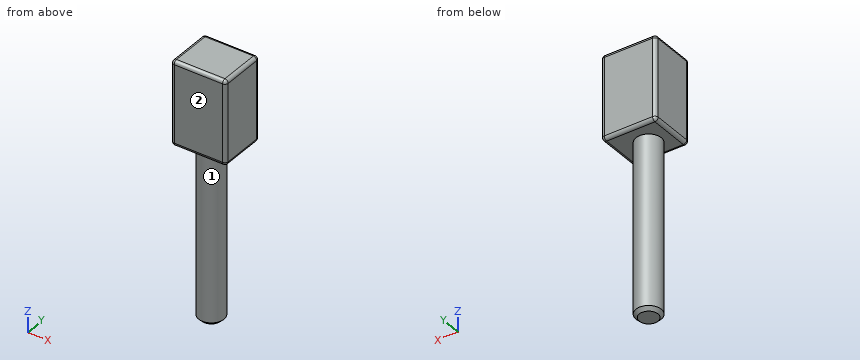
from build123d import *

# Parameters (mm, degrees)
F0_W     = 83.694592
F0_H     = 71.509171
F1_DEPTH = 128.27
F2_R     = 5.08
F3_R     = 19.259612
F4_DEPTH = 263.398
F5_SIZE  = 5.08


with BuildPart() as f1:
    # F0 (on Top) → F1 (new body)
    with BuildSketch(Plane.XY):
        with Locations((3.848031, 2.405015)):
            Rectangle(F0_W, F0_H)
    extrude(amount=F1_DEPTH)

    # F2
    f2_edges = [f1.edges().sort_by_distance(p)[0] for p in [
        (45.695327, 38.159601, 64.135),
        (-37.999265, 38.159601, 64.135),
        (3.848031, 38.159601, 0),
        (3.848031, 38.159601, 128.27),
        (3.848031, -33.34957, 128.27),
        (45.695327, 2.405016, 128.27),
        (-37.999265, 2.405016, 128.27),
        (45.695327, -33.34957, 64.135),
        (45.695327, 2.405016, 0),
        (3.848031, -33.34957, 0),
        (-37.999265, 2.405016, 0),
        (-37.999265, -33.34957, 64.135),
    ]]
    fillet(f2_edges, radius=F2_R)

    # F3 (on Top) → F4 (join)
    with BuildSketch(Plane.XY):
        Circle(F3_R)
    extrude(amount=-F4_DEPTH)

    # F5
    f5_edges = [f1.edges().sort_by_distance(p)[0] for p in [
        (-19.259612, 0, -263.398),
    ]]
    chamfer(f5_edges, length=F5_SIZE)


solid = f1.part
Build history of the part. All positions in model axes, mm. Face numbers are marked on the shaded views. A direction names the side the tool comes from. Give positions to 0.01 mm unless a question says otherwise; leave off trailing zeros. Order: outer loops, then holes, each group sorted by start corner. A loop starts at its lowest first (then second) coordinate and runs counter-clockwise, first axis right, second up. Notation, with made-up numbers: M 84,-27.5 L 96,-27.5 A31 cw 96,1.5 Z; hole C -17,-5 d2. An arc over 180 degrees is marked long. Put each result on its own line as item: value.
Item 1: Wall check: probe 1 along Z at (x, y) = (12, -16); probe 2 along Y at (x, z) = (13, -109); probe 3 along X at (y, z) = (0.5, -196). Give the ranges that are in metal, low to high.
Results are:
probe 1: 0 to 128.27
probe 2: -14.21 to 14.21
probe 3: -19.25 to 19.25
Item 2: Cut at A-A on y = 0. Write the cut outline in (x, z).
Results are:
outline: M -38,5.08 A5.08 ccw -32.92,0 L -19.26,0 L -19.26,-258.32 L -14.18,-263.4 L 14.18,-263.4 L 19.26,-258.32 L 19.26,0 L 40.62,0 A5.08 ccw 45.7,5.08 L 45.7,123.19 A5.08 ccw 40.62,128.27 L -32.92,128.27 A5.08 ccw -38,123.19 Z
Item 3: Cut at C-C on x = 27.5. Write the cut outline in (y, z), then the cut area to 3 significant figures.
Results are:
outline: M -33.35,5.08 A5.08 ccw -28.27,0 L 33.08,0 A5.08 ccw 38.16,5.08 L 38.16,123.19 A5.08 ccw 33.08,128.27 L -28.27,128.27 A5.08 ccw -33.35,123.19 Z
area: 9,150 mm2
Item 4: Drop flat-ended pins along their axis: pin 1 Ø4 at (x, y) = (1.5, -20) entering from -Z; pin 2 Ø5 at (y, z) = (-24, -30.5) entering from +X; pin 3 Ø2 at (x, y) = (-9, 15) entering from -Z; pin 4 Ø5 at (x, y) = (36.5, -24) entering from -Z. Give the stop position or say it passes through.
Results are:
pin 1: z = -259.52
pin 2: through
pin 3: z = -261.08
pin 4: z = 0
Item 5: Which spindle directions (+Z, -Z, +X, -X, +Y, -Y) get a long thin tool onto all of the face, cutting with end or side? Do the marked faces 1 and 2. Say none if no direction does.
Results are:
face 1: -Z
face 2: +Z, -Z, +X, -X, -Y
Item 6: Cut at D-D on z = -196.5. Write the cut outline in (x, y), then the cut area to 3 significant figures.
Results are:
outline: C 0,0 d38.52
area: 1,170 mm2
Item 7: Cut at B-B on x = 0. Write the cut outline in (y, z), then the cut area to 3 significant figures.
Results are:
outline: M -33.35,5.08 A5.08 ccw -28.27,0 L -19.26,0 L -19.26,-258.32 L -14.18,-263.4 L 14.18,-263.4 L 19.26,-258.32 L 19.26,0 L 33.08,0 A5.08 ccw 38.16,5.08 L 38.16,123.19 A5.08 ccw 33.08,128.27 L -28.27,128.27 A5.08 ccw -33.35,123.19 Z
area: 19,300 mm2
